Source: CAD feature listing. Evaluate the final solid. Frame: model axes, mm. Coordinates: 2 decimals unless noted, no trailing zeros. One line per question, with ' | ' between items. Start each with the question number.
1. Pin query (flat end, axial travel): P1, Ø8, axis at x = 45, z = -29, coming from the +Y side; P2, Ø6.5, axis at x = -45, z = -29, coming from the +Y side; P3, Ø6, axis at x = 15, z = 61, coming from the +Y side. Return the tip coordinate at first contact, or that it passes through.
2. Section query A-A, the plane y = -3.5. State how many separate pieces and enclosed holes the cut face has, and give its area (3 significant figures).
3. Ray query, probe 1 along X at (y, z) = (-7.5, 1); probe 2 along Y at (x, z) = (-6, -92); probe 3 along Y at (x, z) = (-47, -2.5). Return the intervals inside material, ascending.
4. Mould query, pull axis Z, two halves, no side actions, for faces 1 (the conical face through (-15.37, -6.66, 88.184)), 2 (the flat face through (-1, -4, 181)), 3 (the flat face through (-60, -4, 3)). Classes: pulls with the +Z half, pulls with the -Z half, needs draft (parallel to the pull), parting line crosses it, or undercut.
```python
from build123d import *

# Parameters (mm, degrees)
ESQUISSE1_W             = 120
ESQUISSE1_H             = 362
BOSS_EXTRU_1_DEPTH      = 8.5
ESQUISSE2_R             = 2.5
ESQUISSE2_R_2           = 1.5
ENL_V_MAT_EXTRU_1_DEPTH = 9.5
CHANFREIN1_SIZE         = 7


with BuildPart() as part:
    # Esquisse1 → Boss.-Extru.1 (new body)
    with BuildSketch(Plane(origin=(0, 0, 0), x_dir=(1, 0, 0), z_dir=(0, 1, 0))):
        Rectangle(ESQUISSE1_W, ESQUISSE1_H)
    extrude(amount=-BOSS_EXTRU_1_DEPTH)

    # Esquisse2 → Enlèv. mat.-Extru.1 (cut, through all)
    with BuildSketch(Plane(origin=(0, 0, 0), x_dir=(1, 0, 0), z_dir=(0, 1, 0))):
        with Locations((-45, 89)):
            Circle(ESQUISSE2_R)
        with Locations((-45, 119)):
            Circle(ESQUISSE2_R_2)
        with Locations((15, 119)):
            Circle(ESQUISSE2_R_2)
        with Locations((-15, 89)):
            Circle(ESQUISSE2_R)
        with Locations((15, 89)):
            Circle(ESQUISSE2_R)
        with Locations((45, 89)):
            Circle(ESQUISSE2_R)
        with Locations((-15, 59)):
            Circle(ESQUISSE2_R)
        with Locations((15, 59)):
            Circle(ESQUISSE2_R)
        with Locations((45, 59)):
            Circle(ESQUISSE2_R)
        with Locations((-15, 29)):
            Circle(ESQUISSE2_R)
        with Locations((15, 29)):
            Circle(ESQUISSE2_R)
        with Locations((45, 29)):
            Circle(ESQUISSE2_R)
        with Locations((-15, -1)):
            Circle(ESQUISSE2_R)
        with Locations((15, -1)):
            Circle(ESQUISSE2_R)
        with Locations((45, -1)):
            Circle(ESQUISSE2_R)
        with Locations((-15, -31)):
            Circle(ESQUISSE2_R)
        with Locations((15, -31)):
            Circle(ESQUISSE2_R)
        with Locations((45, -31)):
            Circle(ESQUISSE2_R)
        with Locations((-15, -61)):
            Circle(ESQUISSE2_R)
        with Locations((15, -61)):
            Circle(ESQUISSE2_R)
        with Locations((45, -61)):
            Circle(ESQUISSE2_R)
        with Locations((-15, -91)):
            Circle(ESQUISSE2_R)
        with Locations((15, -91)):
            Circle(ESQUISSE2_R)
        with Locations((45, -91)):
            Circle(ESQUISSE2_R)
        with Locations((-15, -121)):
            Circle(ESQUISSE2_R)
        with Locations((15, -121)):
            Circle(ESQUISSE2_R)
        with Locations((45, -121)):
            Circle(ESQUISSE2_R)
        with Locations((-45, 59)):
            Circle(ESQUISSE2_R)
        with Locations((-45, 29)):
            Circle(ESQUISSE2_R)
        with Locations((-45, -1)):
            Circle(ESQUISSE2_R)
        with Locations((-45, -31)):
            Circle(ESQUISSE2_R)
        with Locations((-45, -61)):
            Circle(ESQUISSE2_R)
        with Locations((-45, -91)):
            Circle(ESQUISSE2_R)
        with Locations((-45, -121)):
            Circle(ESQUISSE2_R)
    extrude(amount=-ENL_V_MAT_EXTRU_1_DEPTH, mode=Mode.SUBTRACT)

    # Chanfrein1
    chanfrein1_edges = [part.edges().sort_by_distance(p)[0] for p in [
        (12.5, 0, 31),
        (42.5, 0, 31),
        (12.5, 0, 1),
        (-17.5, 0, 1),
        (42.5, 0, -29),
        (12.5, 0, -29),
        (-47.5, 0, 121),
        (-47.5, 0, -89),
        (12.5, 0, 121),
        (-17.5, 0, 121),
        (42.5, 0, 91),
        (12.5, 0, 91),
        (-17.5, 0, 61),
        (12.5, 0, 61),
        (42.5, 0, 61),
        (-17.5, 0, 91),
        (-47.5, 0, 31),
        (-47.5, 0, 61),
        (-47.5, 0, 91),
        (42.5, 0, 121),
        (-47.5, 0, -59),
        (-47.5, 0, -29),
        (-47.5, 0, 1),
        (-17.5, 0, -89),
        (12.5, 0, -89),
        (42.5, 0, -89),
        (-17.5, 0, -29),
        (42.5, 0, -59),
        (12.5, 0, -59),
        (-17.5, 0, -59),
        (42.5, 0, 1),
        (-17.5, 0, 31),
    ]]
    chamfer(chanfrein1_edges, length=CHANFREIN1_SIZE)


solid = part.part
```
Taken from the geometry:
1) P1: y = -5.5 | P2: y = -6.25 | P3: y = -6.5
2) separate pieces: 1 | enclosed holes: 34 | area: 39,800 mm^2
3) probe 1: -60 to -47.5, -42.5 to -17.5, -12.5 to 12.5, 17.5 to 42.5, 47.5 to 60 | probe 2: -8.5 to -0.01 | probe 3: -8.5 to -5.47
4) face 1: undercut | face 2: pulls with the +Z half | face 3: needs draft
